Here's how the part is built. I have some questions about the finished solid (model axes, mm). Face numbers are marked on the shaded views. A direction names the side the tool comes from. Round coordinates to 2 decimals unless told otherwise and drop trailing zeros. Write each loop counter-clockwise with the first axis right and the second up, starting at its lowest first coordinate (ties: lowest second). Pieces come first, ordered by that corner, then holes. Notation, with made-up numbers: M -16.75,4.25 L 40.25,4.25 A23 ccw 40.25,17.25 Z; hole C -14,68.25 d4. An arc over 180 degrees is marked long. Write item = value, one per line. Start each with the question number.
(1) On a 3-axis mill with a long thin cutter (end or side, diameter ignored), from which of +Z, -Z, +X, -X, +Y, -Y can I reach the whole of each face in a straight line? I mean the marked faces 1, 2 and 3. Say none if no direction works.
(2) Will these pins go through, and if not, where does the flat tip stop? pin 1 Ø3.5 at (y, z) = (9.5, 11) entering from +X; pin 2 Ø19 at (y, z) = (10, 50) entering from +X; pin 3 Ø2 at (y, z) = (2, 35) entering from -X; pin 4 Ø6 at (x, y) = (5, 16.5) entering from -Z.
(3) I want a section at A-A (x = 29.5). List the corners of the cut face in (y, z) for me.
(4) I need wall thicknesses on line 1 along Z through (x, y) = (20.5, 5); line 2 along Z through (x, y) = (5, 10.5); line 3 along Y through (x, z) = (2, 50). Which ranges of each line are inside material? Lowest first, please.
(5) I want a section at D-D (y = 31). List the corners of the cut face in (x, z) for me, and give its area (3 significant figures).
(6) I want a section at B-B (z = 30). List the corners of the cut face in (x, y) for me, and give its area (3 significant figures).
(7) I want a section at C-C (x = 2). Give the number of separate pieces and of enclosed holes in the cut face, and give its area (3 significant figures).
(8) If we mould it in two halves opening along Y, with no side actions, what happens to the marked faces 4, 5 and 6? For each: released by +Y, released by -Y, zero draft, split by the parting line, or undercut.
```python
from build123d import *

# Parameters (mm, degrees)
SALIENTE_EXTRUIR1_DEPTH = 60
CROQUIS2_R              = 2.75
CORTAR_EXTRUIR1_DEPTH   = 35
CROQUIS3_R              = 6
CORTAR_EXTRUIR2_DEPTH   = 28
CORTAR_EXTRUIR3_REACH   = 80.702
CROQUIS4_R              = 6.25
CROQUIS5_R              = 10
CORTAR_EXTRUIR4_DEPTH   = 14
REDONDEO1_R             = 10
REDONDEO2_R             = 10
REDONDEO5_R             = 25


with BuildPart() as part:
    # Croquis1 → Saliente-Extruir1 (new body)
    with BuildSketch(Plane.XY):
        Polygon((0, 0), (0, 7), (-1, 7), (-1, 13), (0, 13), (0, 20), (14, 20), (14, 37), (34, 37), (34, 0), align=None)
    extrude(amount=SALIENTE_EXTRUIR1_DEPTH)

    # Croquis2 → Cortar-Extruir1 (cut)
    with BuildSketch(Plane(origin=(34, 0, 0), x_dir=(0, 0, -1), z_dir=(1, 0, 0))):
        with Locations((-50, 10)):
            Circle(CROQUIS2_R)
        with Locations((-10, 10)):
            Circle(CROQUIS2_R)
    extrude(amount=-CORTAR_EXTRUIR1_DEPTH, mode=Mode.SUBTRACT)

    # Croquis3 → Cortar-Extruir2 (cut)
    with BuildSketch(Plane(origin=(34, 0, 0), x_dir=(0, 0, -1), z_dir=(1, 0, 0))):
        with Locations((-50, 10)):
            Circle(CROQUIS3_R)
        with Locations((-10, 10)):
            Circle(CROQUIS3_R)
    extrude(amount=-CORTAR_EXTRUIR2_DEPTH, mode=Mode.SUBTRACT)

    # Croquis4 → Cortar-Extruir3 (cut, up to next)
    with BuildSketch(Plane(origin=(34, 0, 0), x_dir=(0, 0, -1), z_dir=(1, 0, 0)), mode=Mode.PRIVATE) as cortar_extruir3_sk1:
        with Locations((-30, 26)):
            Circle(CROQUIS4_R)
    cortar_extruir3_tool1 = extrude(cortar_extruir3_sk1.sketch, amount=-CORTAR_EXTRUIR3_REACH, mode=Mode.PRIVATE) & part.part
    add(cortar_extruir3_tool1.solids().sort_by_distance((34, 26, 30))[0], mode=Mode.SUBTRACT)

    # Croquis5 → Cortar-Extruir4 (cut)
    with BuildSketch(Plane.ZY.offset(-14)):
        with Locations((30, 26)):
            Circle(CROQUIS5_R)
    extrude(amount=CORTAR_EXTRUIR4_DEPTH, mode=Mode.SUBTRACT)

    # Redondeo1
    redondeo1_edges = [part.edges().sort_by_distance(p)[0] for p in [
        (7, 20, 22),
        (7, 20, 38),
    ]]
    fillet(redondeo1_edges, radius=REDONDEO1_R)

    # Redondeo2
    redondeo2_edges = [part.edges().sort_by_distance(p)[0] for p in [
        (17, 0, 60),
        (7, 20, 60),
        (17, 0, 0),
        (7, 20, 0),
    ]]
    fillet(redondeo2_edges, radius=REDONDEO2_R - 0.0001)  # a hair under: the kernel refuses the full size

    # Redondeo5
    redondeo5_edges = [part.edges().sort_by_distance(p)[0] for p in [
        (24, 37, 60),
        (24, 37, 0),
    ]]
    fillet(redondeo5_edges, radius=REDONDEO5_R)


solid = part.part
```
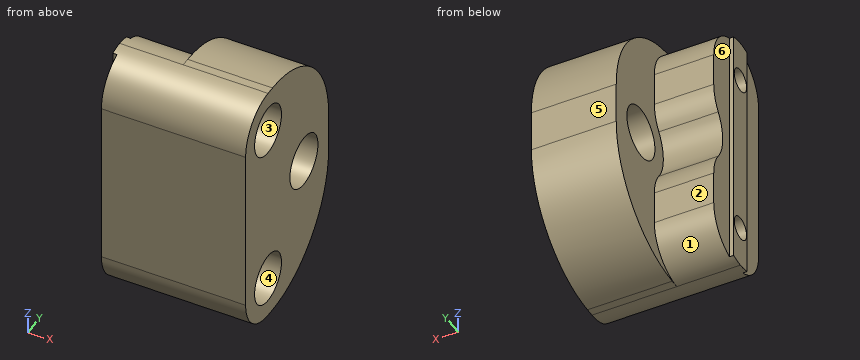
Returned:
q1.face_1 = -Z, -X, +Y
q1.face_2 = +Z, -Z, -X, +Y
q1.face_3 = +X
q2.pin_1 = 6
q2.pin_2 = 34
q2.pin_3 = 0
q2.pin_4 = 0.63
q3.outline = M 0,10 A10 ccw 10,0 L 12,0 A25 ccw 37,25 L 37,35 A25 ccw 12,60 L 10,60 A10 ccw 0,50 Z; hole C 10,10 d12; hole C 10,50 d12; hole C 26,30 d12.5
q4.line_1 = 1.34 to 6.68, 13.32 to 46.68, 53.32 to 58.66
q4.line_2 = 0.01 to 7.3, 12.7 to 47.3, 52.7 to 59.99
q4.line_3 = 0 to 7.25, 12.75 to 20
q5.outline = M 14,8.75 L 34,8.75 L 34,26.25 L 14,26.25 Z; M 14,33.75 L 34,33.75 L 34,51.25 L 14,51.25 Z
q5.area = 700 mm²
q6.outline = M -1,7 L 0,7 L 0,0 L 34,0 L 34,19.75 L 14,19.75 L 14,16 L 0,16 L 0,13 L -1,13 Z; M 14,32.25 L 34,32.25 L 34,37 L 14,37 Z
q6.area = 720 mm²
q7.separate_pieces = 1
q7.enclosed_holes = 2
q7.area = 1,020 mm²
q8.face_4 = undercut
q8.face_5 = released by +Y
q8.face_6 = zero draft
